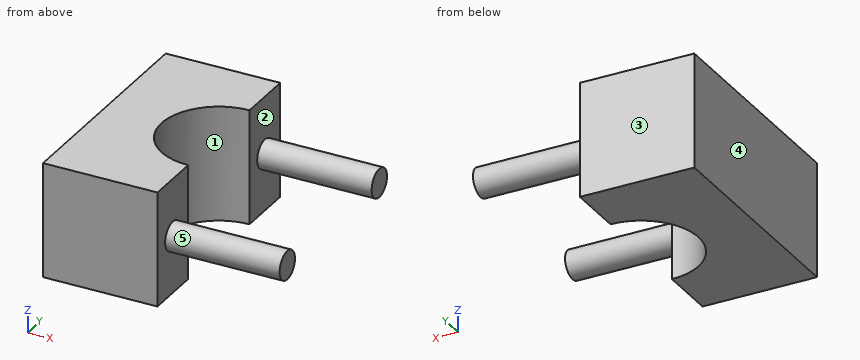
from build123d import *

# Parameters (mm, degrees)
EXTRUDE_1_DEPTH = 20
SKETCH_3_R      = 2.5
EXTRUDE_2_DEPTH = 20


with BuildPart() as part:
    # 草图1 → 凸台-拉伸1 (new body)
    with BuildSketch(Plane.XY):
        with BuildLine():
            Line((0, 20), (0, 10))
            ThreePointArc((0, 10), (-10, 0), (0, -10))
            Line((0, -10), (0, -20))
            Line((0, -20), (-20, -20))
            Line((-20, -20), (-20, 20))
            Line((-20, 20), (0, 20))
        make_face()
    extrude(amount=EXTRUDE_1_DEPTH)

    # 草图3 → 凸台-拉伸2 (add)
    with BuildSketch(Plane(origin=(0, 0, 0), x_dir=(0, 0, -1), z_dir=(1, 0, 0))):
        with Locations(Location((-10, 15, 0), (0, 0, 180))):
            Circle(SKETCH_3_R)
        with Locations(Location((-10, -15, 0), (0, 0, 180))):
            Circle(SKETCH_3_R)
    extrude(amount=EXTRUDE_2_DEPTH)


solid = part.part
Verification items for the finished model (mm, model axes). Face numbers are marked on the shaded views. A direction names the side the tool comes from. Give positions to 0.01 mm unless a question says otherwise; leave off trailing zeros. Write each loop counter-clockwise with the first axis right and the second up, starting at its lowest first coordinate (ties: lowest second). Pieces come first, ordered by that corner, then holes.
(1) Gauge pin test, flat ends, axial feed: pin 1 (5 mm diameter, centred on y = -14.5, z = 2, fed in from +X); pin 2 (2 mm diameter, centred on x = 2, z = 7, fed in from +Y); pin 3 (10 mm diameter, centred on x = 14.5, z = 8.5, fed in from -Y); pin 4 (8 mm diameter, centred on x = 11.5, z = 17.5, fed in from +Y). Record the tip position at first contact, or that the pin passes through.
(2) Access from +Z, -Z, +X, -X, +Y, -Y to the whole of each face (thin tool, end or side, straight path). Record for the marked faces 1 and 2.
(3) Cross-section at A-A (x = -6.5). Enter the section's corners in (y, z).
(4) Cross-section at B-B (z = 10). Enter the section's corners in (x, y).
(5) Cross-section at D-D (z = 6). Enter the section's corners in (x, y).
(6) Mould release check, pull along Y, two halves, no side actions. Record for the marked faces 3, 4 and 5: +Y half, -Y half, draft (parallel to the pull), parting line (faces both ways), or undercut.
(7) Material ranges on line 1 (X direction, y = 15.5, z = 1.5); line 2 (X direction, y = 0, z = 1); line 3 (Y direction, x = -0.5, z = 14.25), recorded low to high.
(8) Cross-section at C-C (y = 15). Enter the section's corners in (x, z).
Worked out:
1. pin 1: stops at x = 0
1. pin 2: stops at y = 16.5
1. pin 3: stops at y = -17.5
1. pin 4: passes through
2. face 1: +Z, -Z, +X
2. face 2: +X
3. outline: (-20, 0) - (-7.6, 0) - (-7.6, 20) - (-20, 20) - close; (7.6, 0) - (20, 0) - (20, 20) - (7.6, 20) - close
4. outline: (-20, -20) - (0, -20) - (0, -17.5) - (20, -17.5) - (20, -12.5) - (0, -12.5) - (0, -10) arc R10 cw to (0, 10) - (0, 12.5) - (20, 12.5) - (20, 17.5) - (0, 17.5) - (0, 20) - (-20, 20) - close
5. outline: (-20, -20) - (0, -20) - (0, -10) arc R10 cw to (0, 10) - (0, 20) - (-20, 20) - close
6. face 3: +Y half
6. face 4: draft
6. face 5: undercut
7. line 1: x = -20 to 0
7. line 2: x = -20 to -10
7. line 3: y = -20 to -9.99, 9.99 to 20
8. outline: (-20, 0) - (0, 0) - (0, 7.5) - (20, 7.5) - (20, 12.5) - (0, 12.5) - (0, 20) - (-20, 20) - close
